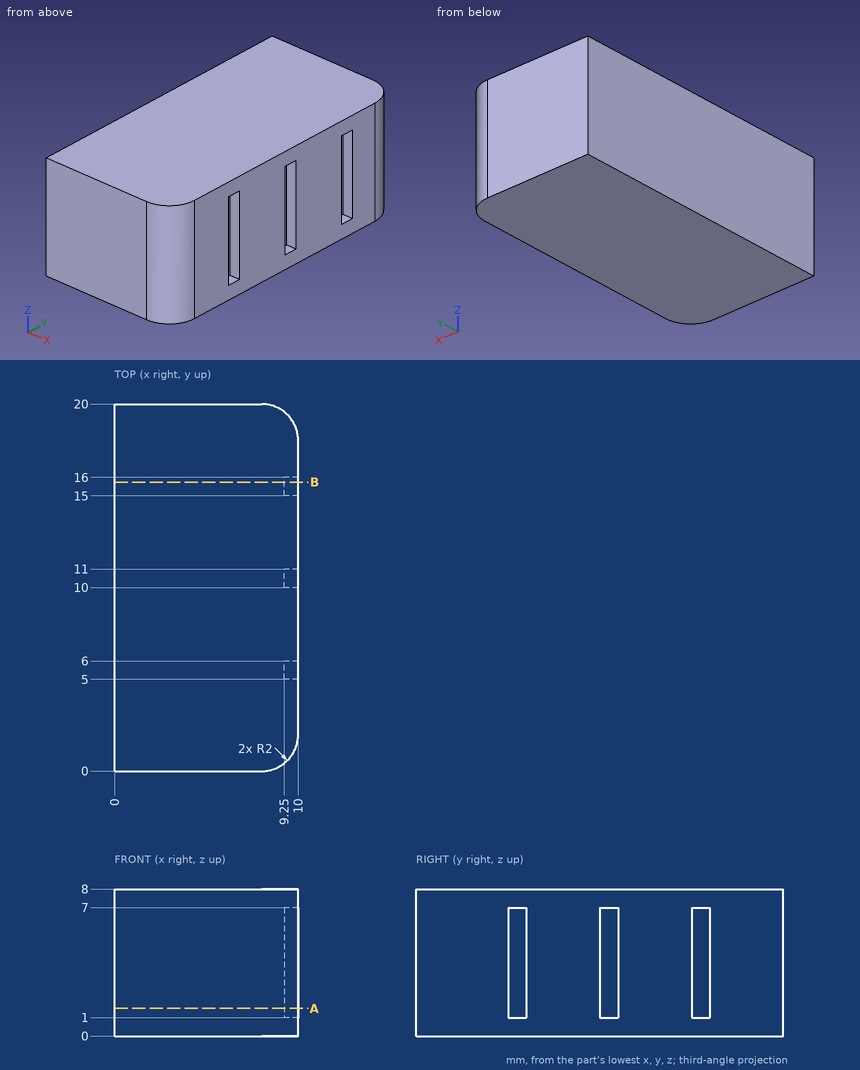
Geometry check sheet. Reference: drawing and pictorial views, mm from the part's lowest x, y, z. Coordinates: 2 decimals unless noted, no trailing zeros. Loops run counter-clockwise (first coordinate to the right, second up) from the corner with the lowest first, then second, coordinate; pieces in that order, holes last. Notation, with made-up numbers: (69, 48) -> (124, 48) arc R26 cw to (124, 78) -> close; hole circle Ø9 at (-22, -25). An arc over 180 degrees is marked (long way). Put each result on its own line as item: value.
1) Thickness scan on line 1 (Y direction, x = 9.75, z = 4.5); line 2 (X direction, y = 5.5, z = 6.5); line 3 (X direction, y = 1.75, z = 7.25). Record the ranges inside material, lowest first.
Result set:
line 1: y = 1.03 to 5, 6 to 10, 11 to 15, 16 to 18.97
line 2: x = 0 to 9.25
line 3: x = 0 to 9.98
2) Gauge pin test, flat ends, axial feed: pin 1 Ø0.8 at (x, z) = (10, 3.5) entering from -Y; pin 2 Ø0.5 at (y, z) = (10.5, 3.5) entering from +X; pin 3 Ø3 at (x, z) = (8.5, 6.5) entering from -Y; pin 4 Ø0.6 at (x, z) = (9.5, 4.5) entering from -Y. Record the tip position at first contact, or that the pin passes through.
Result set:
pin 1: stops at y = 0.8
pin 2: stops at x = 9.25
pin 3: stops at y = 0
pin 4: stops at y = 0.4
3) Cross-section at B-B on y = 15.75. Record the boundary of the cut face in (x, z), plus the area to 3 significant figures.
Result set:
outline: (0, 0) -> (10, 0) -> (10, 1) -> (9.25, 1) -> (9.25, 7) -> (10, 7) -> (10, 8) -> (0, 8) -> close
area: 75.5 mm^2
4) Cross-section at A-A on z = 1.5. Record the boundary of the cut face in (x, y).
Result set:
outline: (0, 0) -> (8, 0) arc R2 ccw to (10, 2) -> (10, 5) -> (9.25, 5) -> (9.25, 6) -> (10, 6) -> (10, 10) -> (9.25, 10) -> (9.25, 11) -> (10, 11) -> (10, 15) -> (9.25, 15) -> (9.25, 16) -> (10, 16) -> (10, 18) arc R2 ccw to (8, 20) -> (0, 20) -> close
